from build123d import *

# Parameters (mm, degrees)
F1_DEPTH  = 112.7125
F2_T      = -1.524
F5_DEPTH  = 225.425
F7_DEPTH  = 225.425
F8_R      = 47.1235523983
F9_DEPTH  = 225.425
F14_W     = 1.27
F14_H     = 1.9164090636
F15_DEPTH = 225.425
F16_R     = 0.508
F17_R     = 6.35
F18_R     = 0.254


with BuildPart() as f1:
    # F0 (on Right) → F1 (new body, symmetric)
    with BuildSketch(Plane.YZ):
        with BuildLine():
            Line((-60.206202515, 18.8091920411), (-18.2712309286, -17.6443226097))
            Line((-18.2712309286, -17.6443226097), (0, 0))
            Line((0, 0), (0, 37.338))
            ThreePointArc((0, 37.338), (-30.365960448, 37.0950138966), (-56.7851466581, 22.1224658109))
            Line((-56.7851466581, 22.1224658109), (-60.206202515, 18.8091920411))
        make_face()
    extrude(amount=F1_DEPTH, both=True)

    # F2
    f2_openings = [f1.faces().sort_by_distance(p)[0] for p in [
        (0, -39.238717, 0.582435),
        (-112.7125, -23.858996, 15.007627),
        (112.7125, -23.858996, 15.007627),
    ]]
    offset(amount=F2_T, openings=f2_openings)

    # F4 (on face) → F5 (join, through all)
    with BuildSketch(Plane(origin=(-112.7125, 0, 0), x_dir=(0, -1, 0), z_dir=(-1, 0, 0))):
        Polygon((57.1348145041, 16.1392751765), (59.0517768379, 17.8056651102), (57.2272137142, 19.5727444541), (55.3102513804, 17.9063545204), align=None)
    extrude(amount=-F5_DEPTH)

    # F6 (on face) → F7 (join, through all)
    with BuildSketch(Plane(origin=(-112.7125, 0, 0), x_dir=(0, -1, 0), z_dir=(-1, 0, 0))):
        Polygon((19.5156410606, -13.2098472516), (17.5986787268, -14.8762371852), (19.4258018197, -16.6406694462), (21.3427641534, -14.9742795125), align=None)
    extrude(amount=-F7_DEPTH)

    # F8 (on face) → F9 (cut, through all)
    with BuildSketch(Plane(origin=(-112.7125, 0, 0), x_dir=(0, -1, 0), z_dir=(-1, 0, 0))):
        with Locations((64.2101801841, -28.1439479334)):
            Circle(F8_R)
    extrude(amount=-F9_DEPTH, mode=Mode.SUBTRACT)

    # F10 (on face) + F11 (on face) + F12 (on face) + F13 (on face) + F14 (on face) → F15 (join, through all)
    with BuildSketch(Plane(origin=(-112.7125, 0, 0), x_dir=(0, -1, 0), z_dir=(-1, 0, 0))):
        Polygon((15.1320625515, -12.4942536329), (16.0456240979, -13.3764697634), (17.5273234081, -12.0884482036), (16.4906753924, -11.0873688514), align=None)
    with BuildSketch(Plane(origin=(-112.7125, 0, 0), x_dir=(0, -1, 0), z_dir=(-1, 0, 0))):
        Polygon((15.577113846, -10.2051527209), (17.5273234081, -12.0884482036), (18.4095395386, -11.1748866572), (16.4593299765, -9.2915911745), align=None)
    with BuildSketch(Plane(origin=(-112.7125, 0, 0), x_dir=(0, -1, 0), z_dir=(-1, 0, 0))):
        Polygon((53.7593727252, 19.4083719627), (55.676335059, 21.0747618964), (54.7640534971, 21.9583015683), (52.8470911634, 20.2919116347), align=None)
    with BuildSketch(Plane(origin=(-112.7125, 0, 0), x_dir=(0, -1, 0), z_dir=(-1, 0, 0))):
        Polygon((4.9915293861, -2.7016545845), (5.9050909325, -3.583870715), (7.2637037735, -2.1769859335), (8.1772653199, -3.059202064), (9.0594814504, -2.1456405176), (7.2323583575, -0.3812082566), align=None)
    with BuildSketch(Plane(origin=(-112.7125, 0, 0), x_dir=(0, -1, 0), z_dir=(-1, 0, 0))):
        Polygon((1.524, 23.3097989494), (1.524, 22.0397989494), (4.7498, 22.0397989494), (4.7498, 24.5797989494), (3.4798, 24.5797989494), (3.4798, 23.3097989494), align=None)
        with Locations((4.1148, 35.8250034812)):
            Rectangle(F14_W, F14_H)
    extrude(amount=-F15_DEPTH)

    # F16
    f16_edges = [f1.edges().sort_by_distance(p)[0] for p in [
        (0, -18.271231, -17.644323),
        (0, -60.206203, 18.809192),
        (0, 0, 37.338),
    ]]
    fillet(f16_edges, radius=F16_R)

    # F17
    f17_edges = [f1.edges().sort_by_distance(p)[0] for p in [
        (0, -1.524, 0.6469),
        (0, 0, 0),
    ]]
    fillet(f17_edges, radius=F17_R)

    # F18
    f18_edges = [f1.edges().sort_by_distance(p)[0] for p in [
        (0, -19.515641, -13.209847),
        (0, -55.641079, 18.193938),
    ]]
    fillet(f18_edges, radius=F18_R)


solid = f1.part
Work out the finished part from the listing and answer in its coordinate system (mm). A direction names the side the tool comes from. Round coordinates to 2 decimals unless told otherwise and drop trailing zeros. Write each loop counter-clockwise with the first axis right and the second up, starting at its lowest first coordinate (ties: lowest second). Pieces come first, ordered by that corner, then holes.
1) A cutting plane is placed at B-B (y = -12). Give the vertices of the cut face in (x, z), plus the area to 3 significant figures.
2) A cutting plane is placed at A-A (z = 28). Give the vertices of the cut face in (x, y).
3) Straight lines are drawn through the part: line 1 (Y direction, x = 71, z = 23.5); line 2 (Y direction, x = 31, z = -2.5); line 3 (Y direction, x = -68, z = -11.5). For each, find the intervals that lie inside material, in ascending order.
4) A tool of negligible diameter and unlimited length cuts with its end or side. For faces 1 (the flat face through (1.578, -9.895, -9.555)), 2 (the cylindrical face through (1.578, -31.118, 35.303)), from which of +Z, -Z, +X, -X, +Y, -Y can it reach the whole face along a straight path? Write none if from no direction.
5) A cutting plane is placed at D-D (z = -6.5). Give the vertices of the cut face in (x, y).
6) A cutting plane is placed at C-C (y = -44). Give the vertices of the cut face in (x, z).
7) The mould has two halves that part along Y. Classify faces 3 (the flat face through (-112.712, -1, 19)), 4 (the cylindrical face through (1.578, -30.146, 37.153)), 5 (the flat face through (2, -1.524, 30)), 6 (the cylindrical face through (1.58, -0.49, 0.25)): pulls with the +Y half, pulls with the -Y half, needs draft (parallel to the pull), parting line crosses it, or undercut.
8) Given pin 1 Ø3 at (y, z) = (-42.5, 30) entering from +X; pin 2 Ø3.5 at (x, y) = (2.5, -2.5) entering from -Z; pin 3 Ø1 at (x, z) = (-87, -5.5) entering from -Y; pin 4 Ø0.6 at (x, y) = (28, -4) entering from +Z, each flat-ended and moving along its own axis, determine where each tip first touches the part or whether it passes through.
Completed:
1. outline: (-112.71, -11.59) - (112.71, -11.59) - (112.71, -9.47) - (-112.71, -9.47) - close; (-112.71, 37.57) - (112.71, 37.57) - (112.71, 39.09) - (-112.71, 39.09) - close
1. area: 821 mm2
2. outline: (-112.71, -49.71) - (112.71, -49.71) - (112.71, -47.01) - (-112.71, -47.01) - close; (-112.71, -1.52) - (112.71, -1.52) - (112.71, 0) - (-112.71, 0) - close
3. line 1: y = -55.31 to -53.01, -4.75 to -3.48, -1.52 to 0
3. line 2: y = -8.72 to -7.6, -6.95 to -5.19, -4.78 to -2.59
3. line 3: y = -18.1 to -16.09, -14.1 to -11.91
4. face 1: -Z, +X, -X, +Y
4. face 2: +X, -X
5. outline: (-112.71, -8.92) - (112.71, -8.92) - (112.71, -6.73) - (-112.71, -6.73) - close
6. outline: (-112.71, 29.84) - (112.71, 29.84) - (112.71, 31.59) - (-112.71, 31.59) - close
7. face 3: needs draft
7. face 4: parting line crosses it
7. face 5: undercut
7. face 6: pulls with the +Y half
8. pin 1: stops at x = 112.71
8. pin 2: stops at z = -4.1
8. pin 3: stops at y = -8.41
8. pin 4: stops at z = 38.25
